```python
from build123d import *

# Parameters (mm, degrees)
F0_W     = 150
F0_H     = 6.5
F0_R     = 1.778
F1_DEPTH = 6.5


with BuildPart() as f1:
    # F0 (on Top) → F1 (new body)
    with BuildSketch(Plane.XY):
        with Locations((75, 3.25)):
            Rectangle(F0_W, F0_H)
        with Locations((5.5, 3.25)):
            Circle(F0_R, mode=Mode.SUBTRACT)
        with Locations((18.1, 3.25)):
            Circle(F0_R, mode=Mode.SUBTRACT)
        with Locations((30.7, 3.25)):
            Circle(F0_R, mode=Mode.SUBTRACT)
        with Locations((44.075, 3.25)):
            Circle(F0_R, mode=Mode.SUBTRACT)
        with Locations((57.45, 3.25)):
            Circle(F0_R, mode=Mode.SUBTRACT)
        with Locations((70.825, 3.25)):
            Circle(F0_R, mode=Mode.SUBTRACT)
        with Locations((84.2, 3.25)):
            Circle(F0_R, mode=Mode.SUBTRACT)
        with Locations((97.575, 3.25)):
            Circle(F0_R, mode=Mode.SUBTRACT)
        with Locations((110.95, 3.25)):
            Circle(F0_R, mode=Mode.SUBTRACT)
        with Locations((124.325, 3.25)):
            Circle(F0_R, mode=Mode.SUBTRACT)
        with Locations((137.7, 3.25)):
            Circle(F0_R, mode=Mode.SUBTRACT)
    extrude(amount=F1_DEPTH)


solid = f1.part
```
Work out the finished part from the listing and answer in its coordinate system (mm). Coordinates: 2 decimals unless noted, no trailing zeros. Write each loop counter-clockwise with the first axis right and the second up, starting at its lowest first coordinate (ties: lowest second). Pieces come first, ordered by that corner, then holes.
Q1. A cutting plane is placed at B-B, the plane x = 110.95. Give the vertices of the cut face in (y, z).
Q2. Determine the mould class of faces 1 (the face through (19.796, 3.784, 3.204)), 2 (the face through (150, 3, 3)), 3 (the face through (74, 0, 3)), 4 (the face through (0, 3, 3)) for opening direction X: released by +X, released by -X, zero draft, split by the parting line, or undercut.
Q3. Find the intervals of material crossed by line 1 (Y direction, x = 110.95, z = 5.25); line 2 (Y direction, x = 83.5, z = 3.5), in increasing order.
Q4. A cutting plane is placed at A-A, the plane z = 3. State how many separate pieces and enclosed holes the cut face has, then the cut area to 3 significant figures.
Findings below:
1. outline: (0, 0) - (1.47, 0) - (1.47, 6.5) - (0, 6.5) - close; (5.03, 0) - (6.5, 0) - (6.5, 6.5) - (5.03, 6.5) - close
2. face 1: undercut
2. face 2: released by +X
2. face 3: zero draft
2. face 4: released by -X
3. line 1: y = 0 to 1.47, 5.03 to 6.5
3. line 2: y = 0 to 1.62, 4.88 to 6.5
4. separate pieces: 1
4. enclosed holes: 11
4. area: 866 mm2
